Design review of the part shown in the three views and the two pictorial views. Dimensions are in mm from the part's minimum x, y and z. Give positions to 0.01 mm unless a question says otherwise; leave off trailing zeros. Loops run counter-clockwise (first coordinate to the right, second up) from the corner with the lowest first, then second, coordinate; pieces in that order, holes last. Notation, with made-up numbers: (-22, 89) -> (-11, 89) arc R9 cw to (-11, 97) -> close; hole circle Ø1 at (64.5, 54.5). An arc over 180 degrees is marked (long way). One line per question, with ' | ' between items. Start each with the question number.
(1) Consider section B-B (z = 55.5). Write out the cut boundary in (x, y).
(2) Consider section A-A (y = 0.95). Give the number of separate pieces and of enclosed holes in the cut face, and give its area (3 significant figures).
(3) Wall thickness on probe 1 along X at (y, z) = (1.7, 110.5); probe 2 along X at (y, z) = (1.65, 136) (1 decimal); probe 3 along Z at (x, y) = (92.55, 1.5): over which ranges is each line inside the solid? List them lowest first.
(4) Insertion check: P1, Ø1, axis at y = 0.5, z = 68, coming from the -X side; P2, Ø1, axis at x = 141.5, y = 1.5, coming from the +Z side. Each pin has a flat end and moves straight along its axis. Give the tip position at first contact, or say it passes through.
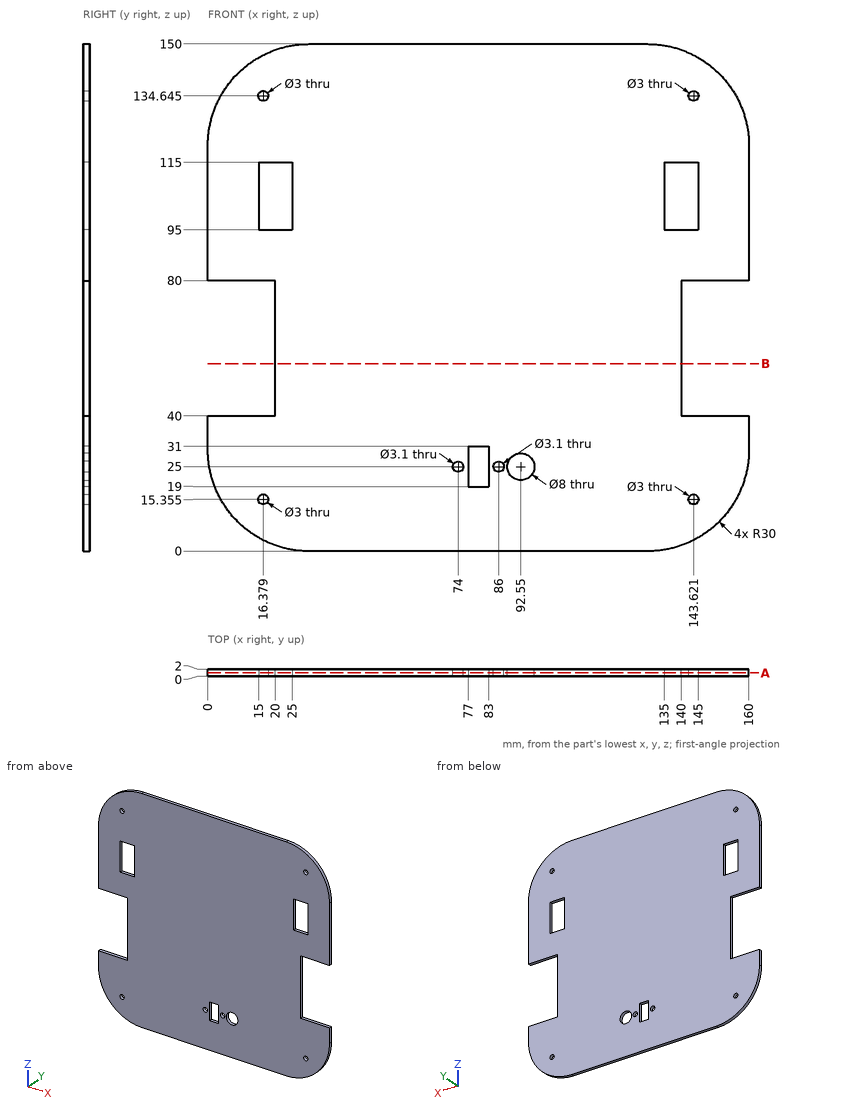
A:
1) outline: (20, 0) -> (140, 0) -> (140, 2) -> (20, 2) -> close
2) separate pieces: 1 | enclosed holes: 10 | area: 21,100 mm^2
3) probe 1: x = 0 to 15, 25 to 135, 145 to 160 | probe 2: x = 4.6 to 15.7, 17 to 143, 144.3 to 155.4 | probe 3: z = 0 to 21, 29 to 150
4) P1: stops at x = 20 | P2: stops at z = 147.91
